```python
from build123d import *

# Parameters (mm, degrees)
SKETCH1_W           = 162.000000477
SKETCH1_H           = 50.000000745
BOSS_EXTRUDE1_DEPTH = 29.999999329
SKETCH2_W           = 145.999998786
SKETCH2_H           = 41.999999434
CUT_EXTRUDE1_DEPTH  = 173.174330807
CUT_EXTRUDE2_DEPTH  = 173.174330807
SKETCH4_W           = 11.999994517
SKETCH4_H           = 6.000000285
CUT_EXTRUDE3_DEPTH  = 173.174330807
CUT_EXTRUDE4_DEPTH  = 171.02352798


with BuildPart() as part:
    # Sketch1 → Boss-Extrude1 (new body)
    with BuildSketch(Plane(origin=(0, 29.999999329, 0), x_dir=(1, 0, 0), z_dir=(0, 1, 0))):
        with Locations((81.000000239, -25.000000373)):
            Rectangle(SKETCH1_W, SKETCH1_H)
    extrude(amount=-BOSS_EXTRUDE1_DEPTH)

    # Sketch2 → Cut-Extrude1 (cut, through all)
    with BuildSketch(Plane.XZ):
        with Locations((80.999999773, 20.999999717)):
            Rectangle(SKETCH2_W, SKETCH2_H)
    extrude(amount=-CUT_EXTRUDE1_DEPTH, mode=Mode.SUBTRACT)

    # Sketch3 → Cut-Extrude2 (cut, through all)
    with BuildSketch(Plane.XY.offset(50.000000745)):
        Polygon((85.776269436, 14.348221011), (85.985377431, 13.061543927), (86.398161948, 11.825070716), (87.003961205, 10.67082677), (87.78706193, 9.628706612), (88.727198541, 8.725699037), (89.800000191, 7.985194214), (90.977698565, 7.426368073), (92.229790986, 7.063695695), (93.523852527, 6.906569004), (94.826348126, 6.959058344), (96.103563905, 7.21980352), (97.322411835, 7.68205151), (98.451323807, 8.333831094), (99.461063743, 9.158260189), (100.325487554, 10.133987293), (101.022191346, 11.23574283), (101.533144712, 12.434989214), (101.845107973, 13.7006687), (101.949997246, 14.999999665), (101.845107973, 16.299331561), (101.533144712, 17.565010116), (101.022191346, 18.764257431), (100.325487554, 19.866012037), (99.461063743, 20.841740072), (98.451323807, 21.666171029), (97.322411835, 22.317949682), (96.103563905, 22.780196741), (94.826348126, 23.040940985), (93.523852527, 23.093432188), (92.229790986, 22.936303169), (90.977698565, 22.573631257), (89.800000191, 22.014804184), (88.727198541, 21.274300292), (87.78706193, 20.371293649), (87.003961205, 19.32917349), (86.398161948, 18.174929544), (85.985377431, 16.938457265), (85.776269436, 15.651779249), align=None)
    extrude(amount=-CUT_EXTRUDE2_DEPTH, mode=Mode.SUBTRACT)

    # Sketch4 → Cut-Extrude3 (cut, through all)
    with BuildSketch(Plane.XY.offset(50.000000745)):
        with Locations((81.000000239, 5.000000238)):
            Rectangle(SKETCH4_W, SKETCH4_H)
    extrude(amount=-CUT_EXTRUDE3_DEPTH, mode=Mode.SUBTRACT)

    # Sketch5 → Cut-Extrude4 (cut, through all)
    with BuildSketch(Plane(origin=(0, 0, 41.999999434), x_dir=(-1, 0, 0), z_dir=(0, 0, -1))):
        Polygon((-70.253565907, 22.780196741), (-71.472413838, 22.317949682), (-72.60132581, 21.666171029), (-73.611065745, 20.841740072), (-74.475489557, 19.866012037), (-75.172193348, 18.764257431), (-75.683146715, 17.565010116), (-75.995109975, 16.299331561), (-76.099999249, 14.999999665), (-75.995109975, 13.7006687), (-75.683146715, 12.434989214), (-75.172193348, 11.23574283), (-74.475489557, 10.133987293), (-73.611065745, 9.158260189), (-72.60132581, 8.333831094), (-71.472413838, 7.68205151), (-70.253565907, 7.21980352), (-68.976350129, 6.959058344), (-67.673847079, 6.906569004), (-66.379792988, 7.063695695), (-65.127700567, 7.426368073), (-63.950002193, 7.985194214), (-62.877193093, 8.725699037), (-61.937060207, 9.628706612), (-61.153959483, 10.67082677), (-60.548167676, 11.825070716), (-60.135371983, 13.061543927), (-59.926263988, 14.348221011), (-59.926263988, 15.651779249), (-60.135371983, 16.938457265), (-60.548167676, 18.174929544), (-61.153959483, 19.32917349), (-61.937060207, 20.371293649), (-62.877193093, 21.274300292), (-63.950002193, 22.014804184), (-65.127700567, 22.573631257), (-66.379792988, 22.936303169), (-67.673847079, 23.093432188), (-68.976350129, 23.040940985), align=None)
    extrude(amount=-CUT_EXTRUDE4_DEPTH, mode=Mode.SUBTRACT)


solid = part.part
```
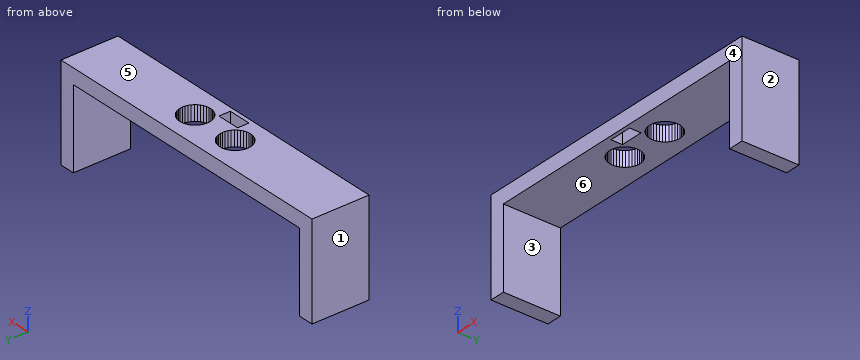
CAD build for the part. Positions are in the model's coordinates, mm. Face numbers are marked on the shaded views. A direction names the side the tool comes from. Coordinates: 2 decimals unless noted, no trailing zeros. Order: outer loops, then holes, each group sorted by start corner. A loop starts at its lowest first (then second) coordinate and runs counter-clockwise, first axis right, second up. Notation, with made-up numbers: M 68,45.5 L 108,45.5 A19 ccw 108,62.5 Z; hole C 9.5,-19.75 d11. An arc over 180 degrees is marked long. Answer as CSV lines item,"result".
1) Cut at B-B (z = 35). List the corners of the cut face in (x, y), then the cut area to 3 significant figures.
Verdict:
outline,"M 0,0 L 8,0 L 8,30 L 0,30 Z; M 154,0 L 162,0 L 162,30 L 154,30 Z"
area,"480 mm2"
2) Cut at C-C (y = 25). List the corners of the cut face in (x, z).
Verdict:
outline,"M 0,0 L 8,0 L 8,42 L 154,42 L 154,0 L 162,0 L 162,50 L 0,50 Z"
3) Cut at D-D (x = 125.5). List the corners of the cut face in (y, z).
Verdict:
outline,"M 0,42 L 30,42 L 30,50 L 0,50 Z"
4) Drill centre lines: L1, parallel to X at y = 17.5, z = 18.5; L2, parallel to X at y = 16.25, z = 42.5; L3, parallel to X at y = 11, z = 46. Where is each one in solid material? Low to high. Write a range as from..to.
Verdict:
L1,"0..8, 154..162"
L2,"0..60.02, 76..85.87, 101.85..162"
L3,"0..60.98, 75.02..86.83, 100.87..162"
5) Flat gauge pin, fed straight in: P1, Ø9, axis at x = 101, y = 21.5, coming from the -Z side. Where does the tip first touch, or does it go through?
Verdict:
P1,"z = 42"
6) 3-axis set-ups, long thin cutter, end or side, ignore diameter. For the marked faces 5 and 6: which of +Z, -Z, +X, -X, +Y, -Y reach the whole face in a straight line?
Verdict:
face 5,"+Z, +X, -X, +Y, -Y"
face 6,"-Z, +Y, -Y"
7) Mould opens along X. For the marked faces 1, 2, 3 and 4 say: released by +X, released by -X, zero draft, split by the parting line, or undercut.
Verdict:
face 1,"released by -X"
face 2,"released by +X"
face 3,"undercut"
face 4,"zero draft"
8) Cut at A-A (y = 5.5). List the corners of the cut face in (x, z).
Verdict:
outline,"M 0,0 L 8,0 L 8,42 L 75,42 L 75,50 L 0,50 Z; M 87,42 L 154,42 L 154,0 L 162,0 L 162,50 L 87,50 Z"
